The model under review builds one solid part; all positions refer to its coordinate system, in mm. A direction names the side the tool comes from. Round coordinates to 2 decimals unless told otherwise and drop trailing zeros. Loops run counter-clockwise (first coordinate to the right, second up) from the corner with the lowest first, then second, coordinate; pieces in that order, holes last. Notation, with made-up numbers: (22, 80.25) -> (72, 80.25) arc R11 ccw to (72, 101.25) -> close; hole circle Ø10 at (-33.5, 31.5). An arc over 180 degrees is marked (long way). Use a Markdown table: item, result. Add a question column.
1) Insertion check: pin 1 (3 mm diameter, centred on x = 3.5, y = -20, fed in from -Z); pin 2 (1.5 mm diameter, centred on y = -2.5, z = 6.5, fed in from +X); pin 3 (1.5 mm diameter, centred on x = 1.5, z = 5, fed in from +Y); pin 4 (18 mm diameter, centred on x = 0, y = 0, fed in from +Z). Each pin has a flat end and moves straight along its axis. Give the tip position at first contact, or say it passes through.
2) Consider section C-C on z = 9. Give the boundary of the cut face in (x, y), plus the area to 3 significant figures.
3) Consider section A-A on x = 0. Give the boundary of the cut face in (y, z).
4) For faces 4 (the cylindrical face through (-14.985, 0.66, 11.507)), 5 (the cylindrical face through (3.47, -15.62, 2.23)), list the 3-axis set-ups (+Z, -Z, +X, -X, +Y, -Y) from which the entire face can be reached by the end or side of a thin tool; tool diameter is ignored.
5) Mouldability with a two-part tool opening along Y and no side actions: class faces 1 (the cylindrical face through (-5.58, -25.14, 5.92)), 2 (the flat face through (11, -11, 12)), 3 (the cylindrical face through (12.54, -9.61, 7.45)) as released by +Y, released by -Y, zero draft, split by the parting line, or undercut.
6) Consider section D-D on z = 3.25. Give the boundary of the cut face in (x, y), plus the area to 3 significant figures.
7) Wall thickness on probe 1 along Y at (x, z) = (0, 11.4); probe 2 along Y at (x, z) = (0, 2.4); probe 3 along X at (y, z) = (-5.5, 1.5): over which ranges is each line inside the solid? List them lowest first.
from build123d import *

# Parameters (mm, degrees)
SKETCH1_R           = 25.75
BOSS_EXTRUDE1_DEPTH = 12
CHAMFER1_SIZE       = 0.6
SKETCH2_R           = 15
CUT_EXTRUDE1_DEPTH  = 13
SKETCH3_R           = 15.8
CUT_EXTRUDE2_DEPTH  = 11
SKETCH4_R           = 16
CUT_EXTRUDE3_DEPTH  = 4
CHAMFER2_SIZE       = 0.5


with BuildPart() as part:
    # Sketch1 → Boss-Extrude1 (new body)
    with BuildSketch(Plane.XY):
        Circle(SKETCH1_R)
    extrude(amount=BOSS_EXTRUDE1_DEPTH)

    # Chamfer1
    chamfer1_edges = [part.edges().sort_by_distance(p)[0] for p in [
        (-25.75, 0, 0),
        (-25.75, 0, 12),
    ]]
    chamfer(chamfer1_edges, length=CHAMFER1_SIZE)

    # Sketch2 → Cut-Extrude1 (cut, through all)
    with BuildSketch(Plane.XY.offset(12)):
        Circle(SKETCH2_R)
    extrude(amount=-CUT_EXTRUDE1_DEPTH, mode=Mode.SUBTRACT)

    # Sketch3 → Cut-Extrude2 (cut)
    with BuildSketch(Plane(origin=(0, 0, 0), x_dir=(-1, 0, 0), z_dir=(0, 0, -1))):
        Circle(SKETCH3_R)
    extrude(amount=-CUT_EXTRUDE2_DEPTH, mode=Mode.SUBTRACT)

    # Sketch4 → Cut-Extrude3 (cut)
    with BuildSketch(Plane(origin=(0, 0, 0), x_dir=(-1, 0, 0), z_dir=(0, 0, -1))):
        Circle(SKETCH4_R)
    extrude(amount=-CUT_EXTRUDE3_DEPTH, mode=Mode.SUBTRACT)

    # Chamfer2
    chamfer2_edges = [part.edges().sort_by_distance(p)[0] for p in [
        (16, 0, 0),
    ]]
    chamfer(chamfer2_edges, length=CHAMFER2_SIZE)


solid = part.part
Result set:
| question | item | result |
|---|---|---|
| 1 | pin 1 | z = 0 |
| 1 | pin 2 | x = 25.69 |
| 1 | pin 3 | y = 25.74 |
| 1 | pin 4 | through |
| 2 | outline | circle Ø51.5 at (0, 0); hole circle Ø31.6 at (0, 0) |
| 2 | area | 1,300 mm2 |
| 3 | outline | (-25.75, 0.6) -> (-25.15, 0) -> (-16.5, 0) -> (-16, 0.5) -> (-16, 4) -> (-15.8, 4) -> (-15.8, 11) -> (-15, 11) -> (-15, 12) -> (-25.15, 12) -> (-25.75, 11.4) -> close; (15, 11) -> (15.8, 11) -> (15.8, 4) -> (16, 4) -> (16, 0.5) -> (16.5, 0) -> (25.15, 0) -> (25.75, 0.6) -> (25.75, 11.4) -> (25.15, 12) -> (15, 12) -> close |
| 4 | face 4 | +Z, -Z |
| 4 | face 5 | -Z |
| 5 | face 1 | split by the parting line |
| 5 | face 2 | zero draft |
| 5 | face 3 | undercut |
| 6 | outline | circle Ø51.5 at (0, 0); hole circle Ø32 at (0, 0) |
| 6 | area | 1,280 mm2 |
| 7 | probe 1 | -25.75 to -15, 15 to 25.75 |
| 7 | probe 2 | -25.75 to -16, 16 to 25.75 |
| 7 | probe 3 | -25.16 to -15.02, 15.02 to 25.16 |
